Can you work these out from the model? Positions are in its coordinate system, mm. Coordinates: 2 decimals unless noted, no trailing zeros. Order: outer loops, then holes, each group sorted by start corner. A loop starts at its lowest first (then second) coordinate and runs counter-clockwise, first axis right, second up. Notation, with made-up numbers: M -37.5,38.25 L -21.5,38.25 A10 ccw -21.5,43.25 Z; hole C 8.25,-20 d11. An arc over 180 degrees is marked long. Answer as a JSON object with one key per item and string values.
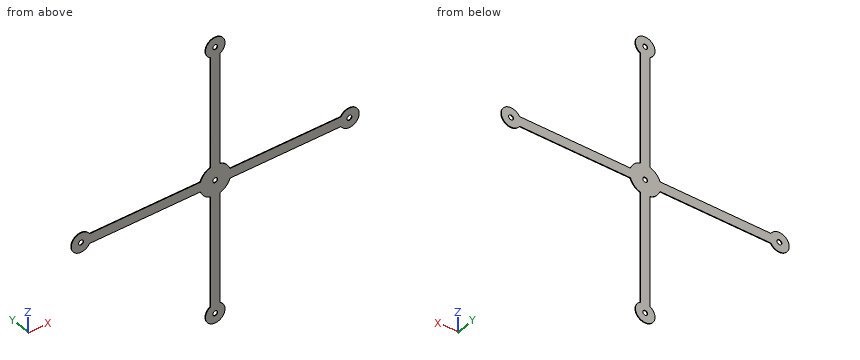
from build123d import *

# Parameters (mm, degrees)
SKETCH1_R           = 1
BOSS_EXTRUDE1_DEPTH = 0.254
SKETCH2_R           = 1
CUT_EXTRUDE1_DEPTH  = 10


with BuildPart() as part:
    # Sketch1 → Boss-Extrude1 (new body)
    with BuildSketch(Plane(origin=(0, 0, 0), x_dir=(1, 0, 0), z_dir=(0, 1, 0))):
        with BuildLine():
            Line((-54.864, 4), (-4.931784667, 4))
            ThreePointArc((-4.931784667, 4), (-4.490128061, 4.490128061), (-4, 4.931784667))
            Line((-4, 4.931784667), (-4, 54.864))
            ThreePointArc((-4, 54.864), (0, 58.864), (4, 54.864))
            Line((4, 54.864), (4, 4.931784667))
            ThreePointArc((4, 4.931784667), (4.490128061, 4.490128061), (4.931784667, 4))
            Line((4.931784667, 4), (54.864, 4))
            ThreePointArc((54.864, 4), (58.864, 0), (54.864, -4))
            Line((54.864, -4), (4.931784667, -4))
            ThreePointArc((4.931784667, -4), (4.490128061, -4.490128061), (4, -4.931784667))
            Line((4, -4.931784667), (4, -54.864))
            ThreePointArc((4, -54.864), (0, -58.864), (-4, -54.864))
            Line((-4, -54.864), (-4, -4.931784667))
            ThreePointArc((-4, -4.931784667), (-4.490128061, -4.490128061), (-4.931784667, -4))
            Line((-4.931784667, -4), (-54.864, -4))
            ThreePointArc((-54.864, -4), (-58.864, 0), (-54.864, 4))
        make_face()
        with Locations((-54.864, 0)):
            Circle(SKETCH1_R, mode=Mode.SUBTRACT)
        with Locations((0, 54.864)):
            Circle(SKETCH1_R, mode=Mode.SUBTRACT)
        with Locations((54.864, 0)):
            Circle(SKETCH1_R, mode=Mode.SUBTRACT)
        with Locations((0, -54.864)):
            Circle(SKETCH1_R, mode=Mode.SUBTRACT)
    extrude(amount=BOSS_EXTRUDE1_DEPTH)

    # Sketch2 → Cut-Extrude1 (cut)
    with BuildSketch(Plane(origin=(0, 0.254, 0), x_dir=(1, 0, 0), z_dir=(0, 1, 0))):
        Circle(SKETCH2_R)
        with BuildLine():
            Line((-2, -51.399898385), (-2, -6.026815079))
            ThreePointArc((-2, -6.026815079), (-3.049552902, -5.569804943), (-4, -4.931784667))
            Line((-4, -4.931784667), (-4, -54.864))
            ThreePointArc((-4, -54.864), (-3.464101615, -52.864), (-2, -51.399898385))
        make_face()
        with BuildLine():
            Line((2, -51.399898385), (2, -6.026815079))
            ThreePointArc((2, -6.026815079), (3.049552902, -5.569804943), (4, -4.931784667))
            Line((4, -4.931784667), (4, -54.864))
            ThreePointArc((4, -54.864), (3.464101615, -52.864), (2, -51.399898385))
        make_face()
        with BuildLine():
            Line((-54.864, 4), (-4.931784667, 4))
            ThreePointArc((-4.931784667, 4), (-5.569804943, 3.049552902), (-6.026815079, 2))
            Line((-6.026815079, 2), (-51.399898385, 2))
            ThreePointArc((-51.399898385, 2), (-52.864, 3.464101615), (-54.864, 4))
        make_face()
        with BuildLine():
            Line((-51.399898385, -2), (-6.026815079, -2))
            ThreePointArc((-6.026815079, -2), (-5.569804943, -3.049552902), (-4.931784667, -4))
            Line((-4.931784667, -4), (-54.864, -4))
            ThreePointArc((-54.864, -4), (-52.864, -3.464101615), (-51.399898385, -2))
        make_face()
        with BuildLine():
            Line((4, 54.864), (4, 4.931784667))
            ThreePointArc((4, 4.931784667), (3.049552902, 5.569804943), (2, 6.026815079))
            Line((2, 6.026815079), (2, 51.399898385))
            ThreePointArc((2, 51.399898385), (3.464101615, 52.864), (4, 54.864))
        make_face()
        with BuildLine():
            Line((-2, 51.399898385), (-2, 6.026815079))
            ThreePointArc((-2, 6.026815079), (-3.049552902, 5.569804943), (-4, 4.931784667))
            Line((-4, 4.931784667), (-4, 54.864))
            ThreePointArc((-4, 54.864), (-3.464101615, 52.864), (-2, 51.399898385))
        make_face()
        with BuildLine():
            Line((54.864, -4), (4.931784667, -4))
            ThreePointArc((4.931784667, -4), (5.569804943, -3.049552902), (6.026815079, -2))
            Line((6.026815079, -2), (51.399898385, -2))
            ThreePointArc((51.399898385, -2), (52.864, -3.464101615), (54.864, -4))
        make_face()
        with BuildLine():
            Line((51.399898385, 2), (6.026815079, 2))
            ThreePointArc((6.026815079, 2), (5.569804943, 3.049552902), (4.931784667, 4))
            Line((4.931784667, 4), (54.864, 4))
            ThreePointArc((54.864, 4), (52.864, 3.464101615), (51.399898385, 2))
        make_face()
    extrude(amount=-CUT_EXTRUDE1_DEPTH, mode=Mode.SUBTRACT)


solid = part.part
Item 1: I'm going to push a flat-ended pin straight in: pin 1 (2 mm diameter, centred on x = 0, z = -24.5, fed in from -Y). Where does the tip first touch, or does it pass through?
Answers follow:
{"pin 1": "stops at y = 0"}
Item 2: Please list where these lines run through material, in increasing order: line 1 (X direction, y = 0.15, z = 0); line 2 (X direction, y = 0.1, z = -51).
Answers follow:
{"line 1": "x = -58.86 to -55.86, -53.86 to -1, 1 to 53.86, 55.86 to 58.86", "line 2": "x = -2 to 2"}
Item 3: I want a section at C-C, the plane z = -15. Write out the boundary of the cut face in (x, y), plus the area to 3 significant figures.
Answers follow:
{"outline": "M -2,0 L 2,0 L 2,0.25 L -2,0.25 Z", "area": "1.02 mm^2"}
Item 4: I want a section at A-A, the plane y = 0.2. Write out the boundary of the cut face in (x, z).
Answers follow:
{"outline": "M -51.4,-2 L -6.03,-2 A6.35 ccw -2,-6.03 L -2,-51.4 A4 ccw long 2,-51.4 L 2,-6.03 A6.35 ccw 6.03,-2 L 51.4,-2 A4 ccw long 51.4,2 L 6.03,2 A6.35 ccw 2,6.03 L 2,51.4 A4 ccw long -2,51.4 L -2,6.03 A6.35 ccw -6.03,2 L -51.4,2 A4 ccw long Z; hole C -54.86,0 d2; hole C 0,-54.86 d2; hole C 0,0 d2; hole C 0,54.86 d2; hole C 54.86,0 d2"}
Item 5: I want a section at B-B, the plane x = -12. Write out the boundary of the cut face in (y, z).
Answers follow:
{"outline": "M 0,-2 L 0.25,-2 L 0.25,2 L 0,2 Z"}
